Study the drawing (mm; zero at the part's minimum x, y, z) and answer. Round coordinates to 2 decimals unless told otherwise and drop trailing zeros. Write each loop counter-clockwise with the first axis right and the second up, starting at its lowest first coordinate (ties: lowest second). Pieces come first, ordered by that corner, then holes.
(1) A cutting plane is placed at B-B, the plane z = 15. Give the vertices of the cut face in (x, y).
(2) Find the intervals of material crossed by probe 1 along Z at (x, y) = (28, 20.5); probe 2 along Y at (x, z) = (15, 27.5), in increasing order.
(3) A cutting plane is placed at A-A, the plane y = 7. Give the vertices of the cut face in (x, z).
(4) A cutting plane is placed at C-C, the plane x = 24. Give the vertices of the cut face in (y, z), and give its area (3 significant figures).
(5) The mould has two halves that part along Z. Classify the marked faces 1, 2, 3 and 4: +Z half, -Z half, draft (parallel to the pull), parting line (faces both ways), or undercut.
(6) Each of these flat-tipped pins is pushed along its axis until it touches: pin 1 Ø10 at (y, z) = (11.5, 26.5) entering from -X; pin 2 Ø5 at (x, z) = (24.5, 25.5) entering from +Y. Where does it stop, or does it pass through?
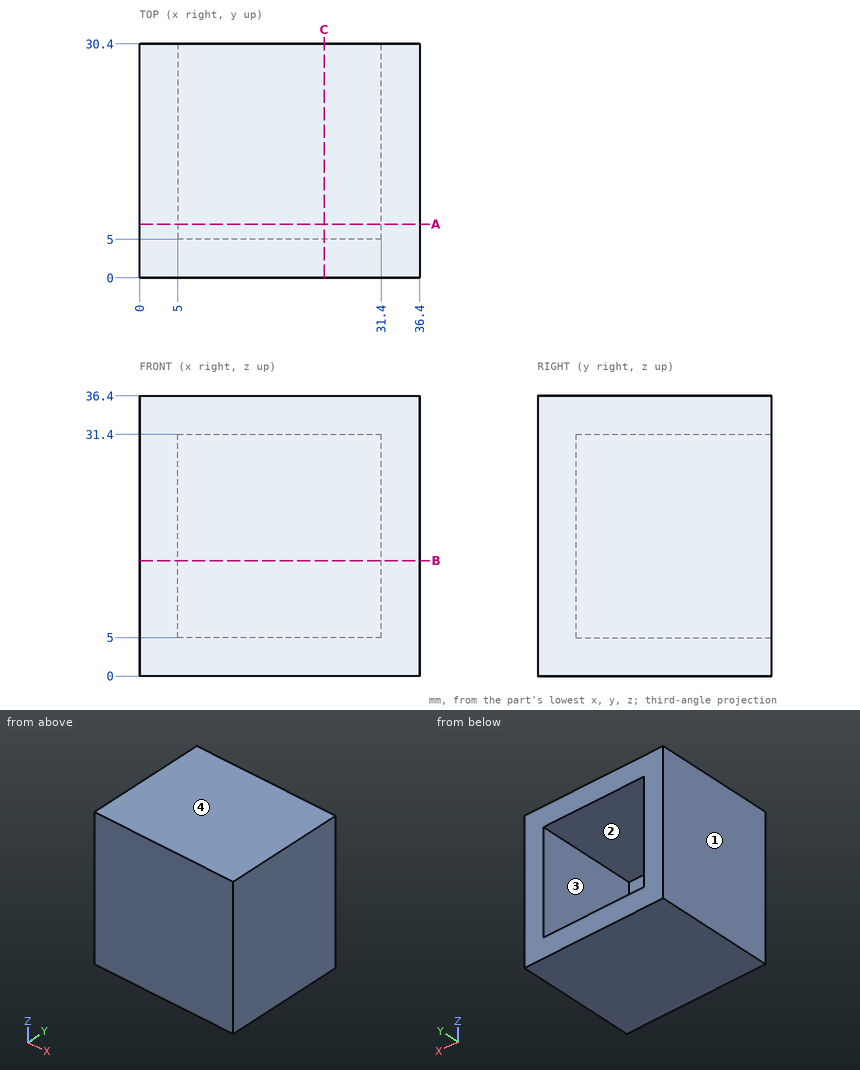
Solutions:
1. outline: (0, 0) - (36.4, 0) - (36.4, 30.4) - (31.4, 30.4) - (31.4, 5) - (5, 5) - (5, 30.4) - (0, 30.4) - close
2. probe 1: z = 0 to 5, 31.4 to 36.4
2. probe 2: y = 0 to 5
3. outline: (0, 0) - (36.4, 0) - (36.4, 36.4) - (0, 36.4) - close; hole (5, 5) - (31.4, 5) - (31.4, 31.4) - (5, 31.4) - close
4. outline: (0, 0) - (30.4, 0) - (30.4, 5) - (5, 5) - (5, 31.4) - (30.4, 31.4) - (30.4, 36.4) - (0, 36.4) - close
4. area: 436 mm2
5. face 1: draft
5. face 2: undercut
5. face 3: undercut
5. face 4: +Z half
6. pin 1: stops at x = 0
6. pin 2: stops at y = 5
